Could you check a few things on this model? Use its own coordinates, in mm. Face numbers are marked on the shaded views. A direction names the side the tool comes from. Give positions to 0.01 mm unless a question says otherwise; leave off trailing zeros. Order: outer loops, then holes, each group sorted by start corner. A loop starts at its lowest first (then second) coordinate and runs counter-clockwise, first axis right, second up. Notation, with made-up numbers: M 49.5,-16.75 L 76.5,-16.75 A18 ccw 76.5,5.25 Z; hole C 51.25,-16 d5. An arc over 180 degrees is marked long. Use a Markdown table: item, result. Add a question column.
Item 1: If we mould it in two halves opening along Z, with no side actions, what happens to the marked faces 4, 5 and 6? For each: released by +Z, released by -Z, zero draft, split by the parting line, or undercut.
Item 2: I'm going to push flat-ended pins straight in: pin 1 Ø6 at (x, z) = (-33, 1) entering from +Y; pin 2 Ø8.5 at (y, z) = (19.8, 19.8) entering from +X; pin 3 Ø6 at (y, z) = (-19.8, -19.8) entering from +X; pin 4 Ø12 at (x, z) = (-32, -18.5) entering from +Y. Where does each tip first touch, or does it pass through?
Item 3: If I drill on L1, parallel to X at y = 24, z = 0 (3 decimals); L2, parallel to X at y = 18.5, z = 3.5; L3, parallel to Y at x = 26, z = 0, over which ranges is the centre line in solid material (lowest first)? Write a range as from..to.
Item 4: Suppose I cut it at B-B on x = -3.5. Write out the boundary of the cut face in (y, z).
Item 5: Suppose I cut it at D-D on x = -38. Write out the boundary of the cut face in (y, z).
Item 6: For the marked faces 1, 2 and 3, which set-ups out of +Z, -Z, +X, -X, +Y, -Y let a thin tool reach every point of the face, with its end or its side?
Item 7: Suppose I cut it at A-A on x = 18.1. Write out the boundary of the cut face in (y, z) (3 decimals), plus the area to 3 significant figures.
Item 8: Suppose I cut it at C-C on z = 0. Count the separate pieces of the cut face and the enclosed holes in it, plus the area to 3 significant figures.
from build123d import *

# Parameters (mm, degrees)
ESQUISSE2_OUTSIDE_W          = 117.85
ESQUISSE2_OUTSIDE_H          = 98.65
ESQUISSE2_OUTSIDE_W_2        = 105
ESQUISSE2_OUTSIDE_H_2        = 66
ENL_V_MAT_EXTRU_1_DEPTH      = 50
ESQUISSE3_R                  = 7.475
ENL_V_MAT_EXTRU_2_DEPTH      = 67
ESQUISSE4_R                  = 3.25
ENL_V_MAT_EXTRU_3_DEPTH      = 80.2
R_P_TITION_CIRCULAIRE1_COUNT = 4
CHANFREIN1_SIZE              = 1


with BuildPart() as part:
    # Esquisse1 → Base-Révolution (revolve)
    with BuildSketch(Plane.XY):
        with BuildLine():
            Line((39.1, 16), (39.1, 20))
            Line((39.1, 20), (36.1, 20))
            Line((36.1, 20), (36.1, 17))
            Line((36.1, 17), (33.5, 17))
            Line((33.5, 17), (33.5, 20))
            Line((33.5, 20), (29.1, 20))
            Line((29.1, 20), (29.1, 35))
            Line((29.1, 35), (7.1, 35))
            Line((7.1, 35), (7.1, 20))
            Line((7.1, 20), (-8.1, 20))
            Line((-8.1, 20), (-12.1, 16))
            Line((-12.1, 16), (-21.738593384, 16))
            ThreePointArc((-21.738593384, 16), (-35.859578061, 21.498655709), (-50.1, 16.317168872))
            Line((-50.1, 16.317168872), (-50.1, 10))
            Line((-50.1, 10), (-47.1, 10))
            Line((-47.1, 10), (-47.1, 13.25))
            Line((-47.1, 13.25), (-43.1, 13.25))
            Line((-43.1, 13.25), (-43.1, 10))
            Line((-43.1, 10), (-29, 10))
            Line((-29, 10), (-28.9, 10.1))
            Line((-28.9, 10.1), (8.2, 10.1))
            Line((8.2, 10.1), (11.1, 13))
            Line((11.1, 13), (36.1, 13))
            Line((36.1, 13), (39.1, 16))
        make_face()
    revolve(axis=Axis((-69, 0, 0), (1, 0, 0)))

    # Esquisse2 outside → Enlèv. mat.-Extru.1 (cut, symmetric)
    with BuildSketch(Plane.XY):
        with Locations((-5.5, 0)):
            Rectangle(ESQUISSE2_OUTSIDE_W, ESQUISSE2_OUTSIDE_H)
        with Locations((-7.5, 0)):
            Rectangle(ESQUISSE2_OUTSIDE_W_2, ESQUISSE2_OUTSIDE_H_2, mode=Mode.SUBTRACT)
    extrude(amount=ENL_V_MAT_EXTRU_1_DEPTH, both=True, mode=Mode.SUBTRACT)

    # Esquisse3 → Enlèv. mat.-Extru.2 (cut, through all)
    with BuildSketch(Plane(origin=(0, 33, 0), x_dir=(-1, 0, 0), z_dir=(0, 1, 0))):
        with Locations((-18.1, 0)):
            Circle(ESQUISSE3_R)
    extrude(amount=-ENL_V_MAT_EXTRU_2_DEPTH, mode=Mode.SUBTRACT)

    # Esquisse4 → Enlèv. mat.-Extru.3 (cut, through all)
    with BuildSketch(Plane(origin=(29.1, 0, 0), x_dir=(0, 0, -1), z_dir=(1, 0, 0))):
        with Locations((19.798989873, -19.798989873)):
            Circle(ESQUISSE4_R)
    enl_v_mat_extru_3 = extrude(amount=-ENL_V_MAT_EXTRU_3_DEPTH, mode=Mode.SUBTRACT)

    # Répétition circulaire1: Enlèv. mat.-Extru.3 ×4 about axis
    r_p_tition_circulaire1_axis = Axis((-69, 0, 0), (1, 0, 0))
    for i in range(1, R_P_TITION_CIRCULAIRE1_COUNT):
        add(enl_v_mat_extru_3.rotate(r_p_tition_circulaire1_axis, i * 360 / R_P_TITION_CIRCULAIRE1_COUNT), mode=Mode.SUBTRACT)

    # Chanfrein1
    chanfrein1_edges = [part.edges().sort_by_distance(p)[0] for p in [
        (39.1, -20, 0),
    ]]
    chamfer(chanfrein1_edges, length=CHANFREIN1_SIZE)


solid = part.part
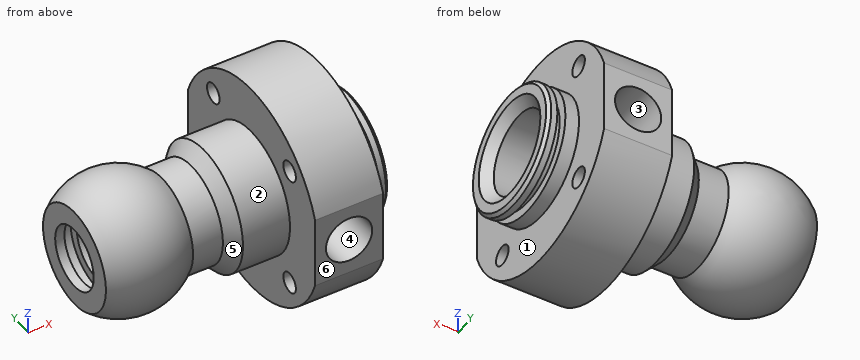
Findings below:
| question | item | result |
|---|---|---|
| 1 | face 4 | undercut |
| 1 | face 5 | split by the parting line |
| 1 | face 6 | zero draft |
| 2 | pin 1 | stops at y = 21.5 |
| 2 | pin 2 | stops at x = 29.1 |
| 2 | pin 3 | passes through |
| 2 | pin 4 | stops at y = 17.16 |
| 3 | L1 | x = 7.1..10.625, 25.575..29.1 |
| 3 | L2 | x = -46.48..-25.72, -9.27..11.5, 24.7..33.5, 36.1..39.1 |
| 3 | L3 | y = -33..-13, 13..33 |
| 4 | outline | C 0,0 d40; hole C 0,0 d20.2 |
| 5 | outline | C 0,0 d42.83; hole C 0,0 d20 |
| 6 | face 1 | +X |
| 6 | face 2 | none |
| 6 | face 3 | +Y, -Y |
| 7 | outline | M -33,-11.662 A35 ccw 33,-11.662 L 33,-7.475 L 10.636,-7.475 A13 cw -10.636,-7.475 L -33,-7.475 Z; M -33,7.475 L -10.636,7.475 A13 cw 10.636,7.475 L 33,7.475 L 33,11.662 A35 ccw -33,11.662 Z; hole C -19.799,-19.799 d6.5; hole C -19.799,19.799 d6.5; hole C 19.799,-19.799 d6.5; hole C 19.799,19.799 d6.5 |
| 7 | area | 2,500 mm^2 |
| 8 | separate pieces | 4 |
| 8 | enclosed holes | 0 |
| 8 | area | 1,420 mm^2 |
